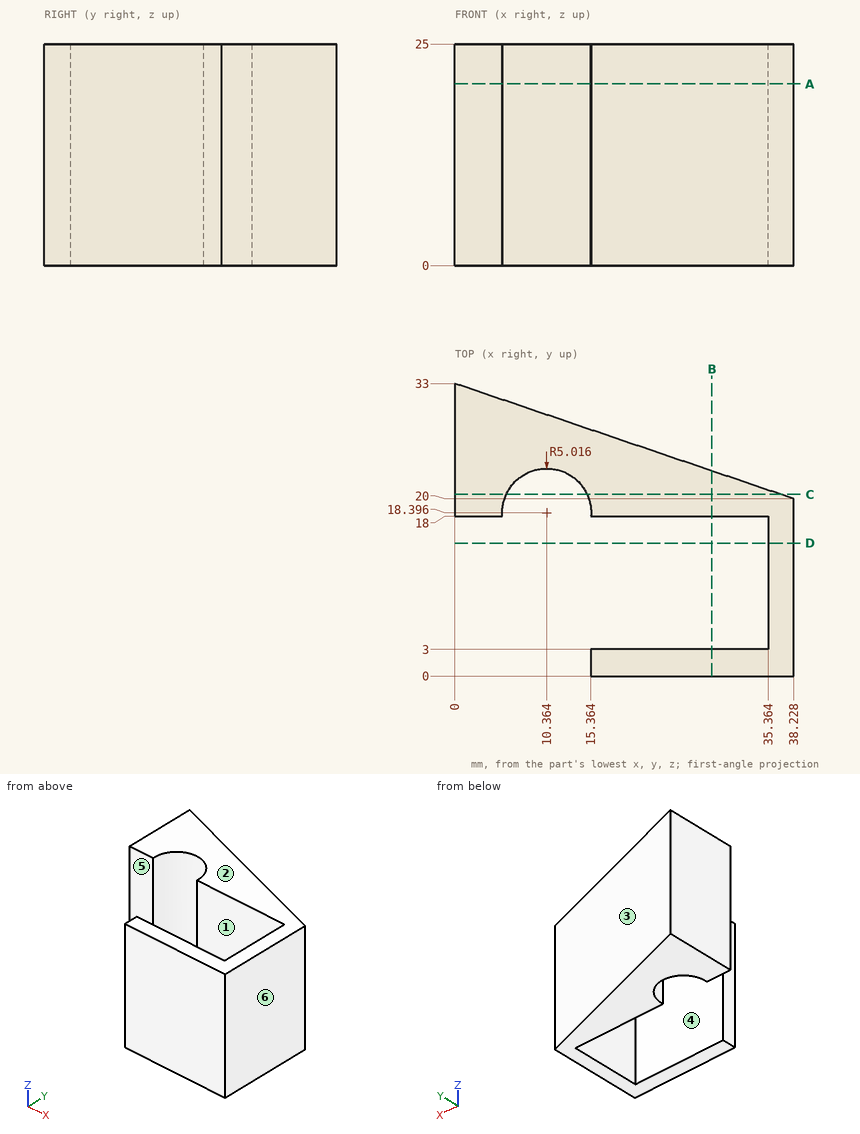
For this review, use the dimensioned drawing (mm, ordinates from the lowest corner) and the shaded views. A direction names the side the tool comes from. Round coordinates to 2 decimals unless told otherwise and drop trailing zeros. Write each loop counter-clockwise with the first axis right and the second up, starting at its lowest first coordinate (ties: lowest second). Pieces come first, ordered by that corner, then holes. Notation, with made-up numbers: M 73.25,4.5 L 77.25,4.5 A21 cw 77.25,33.5 Z; hole C 59,29.25 d11. An arc over 180 degrees is marked long. Use CSV: the item, a comma, the result in double quotes. Start each with the question number.
(1) The part is to be moulded in two halves that separate along Y. For the marked faces 1, 2 and 3, say which applies: +Y half, -Y half, draft (parallel to the pull), parting line (faces both ways), or undercut.
(2) For line 1 along X through (y, z) = (13, 13.5); line 2 along Y through (x, z) = (30.5, 23); line 3 along Y through (x, z) = (19, 10.5), list the stretches that pass through material, from the lowest coordinate up.
(3) We need section A-A, the plane z = 20.5. State the section outline as (x, y) points (1 decimal).
(4) Tool access review of the marked faces 4, 5 and 6: name each direction out of +Z, -Z, +X, -X, +Y, -Y from which nothing blocks a thin tool from reaching the whole face with its end or side.
(5) We need section B-B, the plane x = 29. State the section outline as (y, z) points.
(6) We need section D-D, the plane y = 15. State the section outline as (x, z) points.
(7) Clearance check with flat-ended pins moving along their axes: P1, Ø7.5, axis at y = 10, z = 15, coming from the -X side; P2, Ø5, axis at x = 10, z = 9, coming from the -Y side; P3, Ø10, axis at x = 9, z = 3, coming from the -Y side. State where each tip first meets the part, or that it passes through.
(8) We need section C-C, the plane y = 20.5. State the section outline as (x, z) points, then the cut area to 3 significant figures.
Findings:
1,face 1,"undercut"
1,face 2,"draft"
1,face 3,"+Y half"
2,line 1,"35.36 to 38.23"
2,line 2,"0 to 3, 18 to 22.63"
2,line 3,"0 to 3, 18 to 26.54"
3,outline,"M 0,18 L 5.4,18 A5 cw long 15.4,18 L 35.4,18 L 35.4,3 L 15.4,3 L 15.4,0 L 38.2,0 L 38.2,20 L 0,33 Z"
4,face 4,"+Z, -Z, -X"
4,face 5,"+Z, -Z, -X, -Y"
4,face 6,"+Z, -Z, +X, +Y, -Y"
5,outline,"M 0,0 L 3,0 L 3,25 L 0,25 Z; M 18,0 L 23.14,0 L 23.14,25 L 18,25 Z"
6,outline,"M 35.36,0 L 38.23,0 L 38.23,25 L 35.36,25 Z"
7,P1,"x = 35.36"
7,P2,"y = 22.51"
7,P3,"y = 18"
8,outline,"M 0,0 L 5.81,0 L 5.81,25 L 0,25 Z; M 14.92,0 L 36.76,0 L 36.76,25 L 14.92,25 Z"
8,area,"691 mm^2"
